```python
from build123d import *

# Parameters (mm, degrees)
SKETCH1_W           = 18
SKETCH1_H           = 18
BOSS_EXTRUDE1_DEPTH = 3
SKETCH3_W           = 4.5
SKETCH3_H           = 8
CUT_EXTRUDE1_DEPTH  = 14.076696831
SKETCH6_W           = 18
SKETCH6_H           = 3
BOSS_EXTRUDE3_DEPTH = 15
SKETCH7_W           = 4.5
SKETCH7_H           = 8
CUT_EXTRUDE2_DEPTH  = 28
BOSS_EXTRUDE4_DEPTH = 1
CUT_EXTRUDE3_REACH  = 24.045
SKETCH10_W          = 4.5
SKETCH10_H          = 8


with BuildPart() as part:
    # Sketch1 → Boss-Extrude1 (new body)
    with BuildSketch(Plane(origin=(0, 0, 0), x_dir=(1, 0, 0), z_dir=(0, 1, 0))):
        Rectangle(SKETCH1_W, SKETCH1_H)
    boss_extrude1 = extrude(amount=BOSS_EXTRUDE1_DEPTH)

    # Sketch3 → Cut-Extrude1 (cut, through all)
    with BuildSketch(Plane.XZ):
        with Locations((0, 1)):
            Rectangle(SKETCH3_W, SKETCH3_H)
    extrude(amount=-CUT_EXTRUDE1_DEPTH, mode=Mode.SUBTRACT)

    # Sketch6 → Boss-Extrude3 (add)
    with BuildSketch(Plane(origin=(0, 3, 0), x_dir=(1, 0, 0), z_dir=(0, 1, 0))):
        with Locations((0, 7.5)):
            Rectangle(SKETCH6_W, SKETCH6_H)
    extrude(amount=BOSS_EXTRUDE3_DEPTH)

    # Sketch7 → Cut-Extrude2 (cut, through all)
    with BuildSketch(Plane(origin=(0, 0, -9), x_dir=(-1, 0, 0), z_dir=(0, 0, -1))):
        with Locations((0, 10)):
            Rectangle(SKETCH7_W, SKETCH7_H)
    extrude(amount=-CUT_EXTRUDE2_DEPTH, mode=Mode.SUBTRACT)

    # Sketch9 → Boss-Extrude4 (add)
    with BuildSketch(Plane.ZY.offset(9)):
        Polygon((-6, 18), (9, 3), (-6, 3), align=None)
    boss_extrude4 = extrude(amount=-BOSS_EXTRUDE4_DEPTH)

    # Mirror1: Boss-Extrude1, Boss-Extrude4 across plane
    add(boss_extrude1.mirror(Plane.ZY))
    add(boss_extrude4.mirror(Plane.ZY))

    # Sketch10 → Cut-Extrude3 (cut, up to next)
    with BuildSketch(Plane.XZ, mode=Mode.PRIVATE) as cut_extrude3_sk1:
        with Locations((0, 1)):
            Rectangle(SKETCH10_W, SKETCH10_H)
    cut_extrude3_tool1 = extrude(cut_extrude3_sk1.sketch, amount=-CUT_EXTRUDE3_REACH, mode=Mode.PRIVATE) & part.part
    add(cut_extrude3_tool1.solids().sort_by_distance((0, 0, 1))[0], mode=Mode.SUBTRACT)


solid = part.part
```
Input: part model. Units: mm. Frame: model coordinates. A direction names the side the tool comes from. Coordinates: 2 decimals unless noted, no trailing zeros. Order: outer loops, then holes, each group sorted by start corner. A loop starts at its lowest first (then second) coordinate and runs counter-clockwise, first axis right, second up. Notation, with made-up numbers: (7.5, 17) - (30.5, 17) arc R30 ccw to (30.5, 44) - close; hole circle Ø4 at (-18, 5). An arc over 180 degrees is marked (long way). Return JSON: item names as keys, results as strings.
Q1. Access query for faces 1 (the flat face through (-4, 10, -6)), 2 (the flat face through (0, 14, -8)), 3 (the flat face through (0, 1, 5)). Directions: +Z, -Z, +X, -X, +Y, -Y. A direction counts if a zero-diameter tool reaches every point of the face in a straight line with its end or side. Return the directions, or none.
The answers:
{"face 1": "+Z, +Y", "face 2": "+Z, -Z", "face 3": "+Y, -Y"}
Q2. Cut plane D-D (y = 16.25). Return loops of the section in (x, z), then the cut area to 3 significant figures.
The answers:
{"outline": "(-9, -9) - (9, -9) - (9, -4.25) - (8, -4.25) - (8, -6) - (-8, -6) - (-8, -4.25) - (-9, -4.25) - close", "area": "57.5 mm2"}
Q3. Cut plane C-C (x = -1.25). Return loops of the section in (y, z), then the cut area to 3 significant figures.
The answers:
{"outline": "(0, -9) - (6, -9) - (6, -6) - (3, -6) - (3, -3) - (0, -3) - close; (0, 5) - (3, 5) - (3, 9) - (0, 9) - close; (14, -9) - (18, -9) - (18, -6) - (14, -6) - close", "area": "51.0 mm2"}
Q4. Cut plane A-A (z = 2.75). Return loops of the section in (x, y).
The answers:
{"outline": "(-9, 0) - (-2.25, 0) - (-2.25, 3) - (-8, 3) - (-8, 9.25) - (-9, 9.25) - close; (2.25, 0) - (9, 0) - (9, 9.25) - (8, 9.25) - (8, 3) - (2.25, 3) - close"}
Q5. Ray query, probe 1 along Y at (x, z) = (1.25, -6.75); probe 2 along Z at (x, y) = (0, 1.75); probe 3 along X at (y, z) = (8, -3.75). Return the intervals inside material, ascending.
The answers:
{"probe 1": "y = 0 to 6, 14 to 18", "probe 2": "z = -9 to -3, 5 to 9", "probe 3": "x = -9 to -8, 8 to 9"}
Q6. Cut plane B-B (y = 11). Return loops of the section in (x, z).
The answers:
{"outline": "(-9, -9) - (-2.25, -9) - (-2.25, -6) - (-8, -6) - (-8, 1) - (-9, 1) - close; (2.25, -9) - (9, -9) - (9, 1) - (8, 1) - (8, -6) - (2.25, -6) - close"}
Q7. Draft query along Z for faces 4 (the flat face through (-8.5, 10.6, 1.4)), 5 (the flat face through (-2.25, 1, 1)), 6 (the flat face through (0, 1, -3)), 7 (the flat face through (-2.25, 10, -8)). Return one class per face: +Z half, -Z half, draft (parallel to the pull), parting line (faces both ways), or undercut.
The answers:
{"face 4": "+Z half", "face 5": "undercut", "face 6": "undercut", "face 7": "draft"}
Q8. First-contact query: pin 1 (4.5 mm diameter, centred on x = 1.5, y = 9, fed in from +Z); pin 2 (7.5 mm diameter, centred on x = -3, z = 4, fed in from +Y). Flat tips, straight axial feed; report the tip coordinate or a pass-through.
The answers:
{"pin 1": "stops at z = -6", "pin 2": "stops at y = 3"}
